Autodesk Inventor part; units mm, degrees
ref_plane "YZ Plane" through (0, 0, 0) normal (1, 0, 0) x (0, 1, 0)
ref_plane "XZ Plane" through (0, 0, 0) normal (0, 1, 0) x (-1, 0, 0)
ref_plane "XY Plane" through (0, 0, 0) normal (0, 0, 1) x (1, 0, 0)
sketch "Sketch1" plane through (0, 0, 0) normal (0, 1, 0) x (-1, 0, 0)
  line L0 (0, 0) -> (155, 0)
  line L1 (155, 0) -> (155, -130)
  line L2 (155, -130) -> (0, -130)
  line L3 (0, -130) -> (0, 0)
  dimension "d0" = 130
  dimension "d1" = 155
extrude "Extrusion1" add sketch "Sketch1" along normal blind 60
sketch "Sketch2" plane through (0, 60, 0) normal (0, 1, 0) x (1, 0, 0)
  line L0 (-150, 5) -> (-5, 5)
  line L1 (-5, 5) -> (-5, 125)
  line L2 (-5, 125) -> (-150, 125)
  line L3 (-150, 125) -> (-150, 5)
  line L4 (-155, 0) -> (0, 0)
  line L5 (0, 130) -> (-155, 130)
  line L6 (-155, 130) -> (-155, 0)
  line L7 (0, 0) -> (0, 130)
  point P0 (-77.5, 130)
  dimension "d4" = 5
  dimension "d5" = 5
  dimension "d6" = 5
  dimension "d7" = 5
extrude "Extrusion2" cut sketch "Sketch2" against normal blind 55 contours L3 L2 L1 L0
sketch "Sketch3" plane through (0, 60, 0) normal (0, 1, 0) x (1, 0, 0)
  line L0 (-155, 0) -> (0, 0)
  line L1 (-155, 0) -> (0, 0)
  line L2 (0, 0) -> (0, 130)
  line L3 (0, 130) -> (-155, 130)
  line L4 (-155, 130) -> (-155, 0)
extrude "Extrusion3" add sketch "Sketch3" along normal blind 5
sketch "Sketch4" plane through (0, 65, 0) normal (0, 1, 0) x (1, 0, 0)
  circle A0 centre (-30, 100) radius 5
  line L0 (0, 130) -> (-155, 130)
  line L1 (0, 0) -> (0, 130)
  dimension "d12" = 10
  dimension "d13" = 30
  dimension "d14" = 30
extrude "Extrusion4" cut sketch "Sketch4" against normal blind 5
sketch "Sketch5" plane through (-155, 0, 0) normal (0, 0, 1) x (1, 0, 0)
  circle A0 centre (20, 20) radius 5
  line L0 (0, 0) -> (155, 0)
  line L1 (0, 0) -> (0, 65)
  dimension "d17" = 20
  dimension "d18" = 20
  dimension "d19" = 10
extrude "Extrusion5" cut sketch "Sketch5" against normal blind 20
sketch "Sketch6" plane through (0, 65, 0) normal (0, 1, 0) x (1, 0, 0)
  line L0 (-145, 5) -> (-105, 5)
  line L1 (-105, 5) -> (-105, 125)
  line L2 (-105, 125) -> (-145, 125)
  line L3 (-145, 125) -> (-145, 5)
  line L4 (-155, 130) -> (-155, 0)
  line L5 (0, 130) -> (-155, 130)
  line L6 (-155, 0) -> (0, 0)
  point P0 (-125, 5)
  dimension "d22" = 10
  dimension "d23" = 5
  dimension "d24" = 5
  dimension "d25" = 40
extrude "Extrusion6" cut sketch "Sketch6" against normal blind 5
sketch "Sketch7" plane through (-155, 0, 0) normal (0, 0, 1) x (1, 0, 0)
  circle A0 centre (20, 30) radius 1.5
  circle A1 centre (20, 20) radius 5
  circle A2 centre (20, 20) radius 5
  circle A3 centre (10, 20) radius 1.5
  circle A4 centre (20, 10) radius 1.5
  circle A5 centre (30, 20) radius 1.5
  point P0 (155, 0)
  dimension "d28" = 3
  dimension "d31" = 360
  dimension "d35" = 10
extrude "Extrusion7" cut sketch "Sketch7" against normal blind 5 contours A0 | A3 | A4 | A5
sketch "Sketch8" plane through (0, 65, 0) normal (0, 1, 0) x (1, 0, 0)
  point P0 (0, 0)
sketch "Sketch9" plane through (0, 65, 0) normal (0, 1, 0) x (1, 0, 0)
  point P0 (0, 0)
sketch "Sketch10" plane through (0, 65, 0) normal (0, 1, 0) x (1, 0, 0)
  point P0 (0, 0)
chamfer "Chamfer1" distance 1 angle 45 4 edges at (-126.5, 20, 0) (-136.5, 30, 0) (-136.5, 10, 0) (-146.5, 20, 0)
chamfer "Chamfer3" distance 1 angle 45 4 edges at (-105, 65, -65) (-125, 65, -125) (-145, 65, -65) (-125, 65, -5)
sketch "Sketch12" plane through (-5, 5, -5) normal (0, 0, -1) x (-1, 0, 0)
  line L0 (0, 0) -> (145, 0)
  line L1 (145, 0) -> (115, 0)
  line L2 (115, 0) -> (115, 30)
  line L3 (115, 30) -> (145, 30)
  line L4 (145, 30) -> (145, 0)
  point P0 (-5, -5)
  point P1 (115, 0)
  dimension "d53" = 30
  dimension "d54" = 30
extrude "Extrusion9" add sketch "Sketch12" along normal blind 5
sketch "Sketch13" plane through (-155, 0, 0) normal (0, 0, 1) x (1, 0, 0)
  point P0 (155, 0)
sketch "Sketch14" plane through (-135, 20, -5) normal (0, 0, 1) x (1, 0, 0)
  circle A0 centre (0, 0) radius 5
  point P0 (135, -20)
extrude "Extrusion10" cut sketch "Sketch14" against normal blind 20
chamfer "Chamfer4" distance 1 angle 45 2 edges at (-35, 65, -100) (-140, 20, 0)
chamfer "Chamfer5" distance 3 angle 45 12 edges at (0, 65, -65) (-77.5, 65, 0) (-155, 65, -65) (-77.5, 65, -130) (0, 32.5, 0) (0, 32.5, -130) (-155, 32.5, -130) (-155, 32.5, 0) (0, 0, -65) (-77.5, 0, -130) (-155, 0, -65) (-77.5, 0, 0)
sketch "Sketch15" plane through (0, 65, 0) normal (0, 1, 0) x (1, 0, 0)
  point P0 (0, 0)
sketch "Sketch16" plane through (0, 65, 0) normal (0, 1, 0) x (1, 0, 0)
  point P0 (0, 0)
sketch "Sketch17" plane through (-152, 3, 0) normal (0, 0, 1) x (1, 0, 0)
  point P0 (152, -3)
sketch "Sketch18" plane through (-152, 3, 0) normal (0, 0, 1) x (1, 0, 0)
  point P0 (152, -3)
sketch "Sketch19" plane through (-152, 3, 0) normal (0, 0, 1) x (1, 0, 0)
  point P0 (152, -3)
sketch "Sketch20" plane through (0, 65, 0) normal (0, 1, 0) x (1, 0, 0)
  point P0 (0, 0)
sketch "Sketch21" plane through (-152, 3, 0) normal (0, 0, 1) x (1, 0, 0)
  point P0 (152, -3)
sketch "Sketch22" plane through (0, 65, 0) normal (0, 1, 0) x (1, 0, 0)
  circle A0 centre (-30, 110) radius 1.5
  circle A1 centre (-30, 100) radius 5
  circle A2 centre (-40, 100) radius 1.5
  circle A3 centre (-30, 90) radius 1.5
  circle A4 centre (-20, 100) radius 1.5
  point P0 (0, 0)
  dimension "d66" = 3
  dimension "d67" = 10
  dimension "d70" = 360
sketch "Sketch23" plane through (-152, 3, 0) normal (0, 0, 1) x (1, 0, 0)
  point P0 (152, -3)
extrude "Extrusion11" cut sketch "Sketch22" against normal blind 10 contours A0 | A2 | A3 | A4
chamfer "Chamfer6" distance 1 angle 45 4 edges at (-21.5, 65, -100) (-31.5, 65, -110) (-41.5, 65, -100) (-31.5, 65, -90)
sketch "Sketch24" plane through (-152, 3, 0) normal (0, 0, 1) x (1, 0, 0)
  point P0 (152, -3)
equation "\"BendRadius\" = Thickness"
equation "\"BendReliefWidth\" = Thickness"
equation "\"BendReliefDepth\" = 0.5 * Thickness"
equation "\"CornerReliefSize\" = 4 * Thickness"
equation "\"MinimumRemnant\" = 2 * Thickness"
equation "\"TransitionRadius\" = BendRadius"
equation "\"JacobiRadiusSize\" = BendRadius"
equation "\"GapSize\" = Thickness"
properties part number "Water container"
The listing builds one solid part. Answer for the finished solid, in the listing's coordinates (mm). A direction names the side the tool comes from. Give positions to 0.01 mm unless a question says otherwise; leave off trailing zeros. Order: outer loops, then holes, each group sorted by start corner. A loop starts at its lowest first (then second) coordinate and runs counter-clockwise, first axis right, second up. Notation, with made-up numbers: (25.5, -38) -> (43.5, -38) arc R20 ccw to (43.5, -30) -> close; hole circle Ø5 at (81, -25). An arc over 180 degrees is marked (long way). One line per item, written item: value.
1) Find section B-B, the plane z = -62.5. Determine the outline of the cut face in (x, y), plus the area to 3 significant figures.
Reported:
outline: (-155, 3) -> (-152, 0) -> (-3, 0) -> (0, 3) -> (0, 62) -> (-3, 65) -> (-104, 65) -> (-105, 64) -> (-105, 60) -> (-5, 60) -> (-5, 5) -> (-150, 5) -> (-150, 60) -> (-145, 60) -> (-145, 64) -> (-146, 65) -> (-152, 65) -> (-155, 62) -> close
area: 1,880 mm^2
2) Find the intervals of material crossed by line 1 (Y direction, x = -135, z = -4); line 2 (X direction, y = 62, z = -100); line 3 (Z direction, x = -30, y = 62), in increasing order.
Reported:
line 1: y = 0 to 8.5, 11.5 to 15, 25 to 28.5, 31.5 to 65
line 2: x = -155 to -145, -105 to -41.5, -38.5 to -35, -25 to -21.5, -18.5 to 0
line 3: z = -130 to -111.5, -108.5 to -105, -95 to -91.5, -88.5 to 0
3) A tool of negligible diameter and unlimited length cuts with its end or side. For faces 5 (the flat face through (-79, 5, -66)), 6 (the flat face through (-145, 62, -66)), 7 (the cylindrical face through (-132.693, 15.564, -5.437)), 8 (the flat face through (-76, 0, -64)), 9 (the flat face through (-79, 32, 0)), from which of +Z, -Z, +X, -X, +Y, -Y can it reach the whole face along a straight path? Write none if from no direction.
Reported:
face 5: none
face 6: +Y
face 7: +Z
face 8: +Z, -Z, +X, -X, -Y
face 9: +Z, +X, -X, +Y, -Y
4) Determine the mould class of faces 1 (the flat face through (0, 32, -64)), 2 (the flat face through (-76, 35, -125)), 3 (the flat face through (-155, 32, -66)), 4 (the flat face through (-76, 32, -130)) for opening direction X: pulls with the +X half, pulls with the -X half, needs draft (parallel to the pull), parting line crosses it, or undercut.
Reported:
face 1: pulls with the +X half
face 2: undercut
face 3: pulls with the -X half
face 4: needs draft
5) Find section A-A, the plane x = -46.5. Determine the outline of the cut face in (y, z), plus the area to 3 significant figures.
Reported:
outline: (0, -127) -> (3, -130) -> (62, -130) -> (65, -127) -> (65, -3) -> (62, 0) -> (3, 0) -> (0, -3) -> close; hole (5, -125) -> (60, -125) -> (60, -5) -> (5, -5) -> close
area: 1,830 mm^2
6) Flat-ended cylindrical pins translate along their axes: P1, Ø1.8, axis at x = -135, y = 10, coming from the +Z side; P2, Ø6, axis at x = -30, z = -100, coming from the -Y side; P3, Ø2.5, axis at x = -130.5, z = -8, coming from the +Y side; P4, Ø2.5, axis at x = -144.5, y = 20, coming from the +Z side. Find the tip coordinate at first contact, or state that the pin passes through.
Reported:
P1: stops at z = -5
P2: stops at y = 0
P3: stops at y = 35
P4: stops at z = -0.75
